CAD build for the part. Positions are in the model's coordinates, mm. A direction names the side the tool comes from. Round coordinates to 2 decimals unless told otherwise and drop trailing zeros. Loops run counter-clockwise (first coordinate to the right, second up) from the corner with the lowest first, then second, coordinate; pieces in that order, holes last. Notation, with made-up numbers: M -6,12 L 40,12 A24 ccw 40,46 Z; hole C 70.25,54.25 d1. An arc over 180 degrees is marked long. Use one line per item in the form item = value.
from build123d import *

# Parameters (mm, degrees)
SKETCH1_R           = 2
BOSS_EXTRUDE1_DEPTH = 2
CHAMFER1_SIZE       = 0.3
CUT_EXTRUDE1_DEPTH  = 1.5
CHAMFER2_SIZE       = 0.2
SKETCH3_R           = 1
BOSS_EXTRUDE2_DEPTH = 6
CHAMFER3_SIZE       = 0.2


with BuildPart() as part:
    # Sketch1 → Boss-Extrude1 (new body)
    with BuildSketch(Plane(origin=(0, 0, 0), x_dir=(1, 0, 0), z_dir=(0, 1, 0))):
        with Locations(Location((0, 0, 0), (0, 0, 270))):  # turned: the seam where the file's is
            Circle(SKETCH1_R)
    extrude(amount=BOSS_EXTRUDE1_DEPTH)

    # Chamfer1
    chamfer1_edges = [part.edges().sort_by_distance(p)[0] for p in [
        (0, 2, -2),
    ]]
    chamfer(chamfer1_edges, length=CHAMFER1_SIZE)

    # Sketch2 → Cut-Extrude1 (cut)
    with BuildSketch(Plane(origin=(0, 2, 0), x_dir=(1, 0, 0), z_dir=(0, 1, 0))):
        Polygon((1.154700538, 0), (0.577350269, 1), (-0.577350269, 1), (-1.154700538, 0), (-0.577350269, -1), (0.577350269, -1), align=None)
    extrude(amount=-CUT_EXTRUDE1_DEPTH, mode=Mode.SUBTRACT)

    # Chamfer2
    chamfer2_edges = [part.edges().sort_by_distance(p)[0] for p in [
        (0.866025404, 2, 0.5),
        (0.866025404, 2, -0.5),
        (0, 2, -1),
        (-0.866025404, 2, -0.5),
        (-0.866025404, 2, 0.5),
        (0, 2, 1),
    ]]
    chamfer(chamfer2_edges, length=CHAMFER2_SIZE)

    # Sketch3 → Boss-Extrude2 (add)
    with BuildSketch(Plane.XZ):
        with Locations(Location((0, 0, 0), (0, 0, 90))):  # turned: the seam where the file's is
            Circle(SKETCH3_R)
    extrude(amount=BOSS_EXTRUDE2_DEPTH)

    # Chamfer3
    chamfer3_edges = [part.edges().sort_by_distance(p)[0] for p in [
        (0, -6, -1),
    ]]
    chamfer(chamfer3_edges, length=CHAMFER3_SIZE)


solid = part.part
1. Tool access for faces 5 (the face through (0, -6, 0)), 6 (the face through (-0.86, 1.16, -0.51)), 7 (the face through (-1, 0, 1)): list every direction of +Z, -Z, +X, -X, +Y, -Y with a clear straight run to the whole face (end or side of a thin tool).
Completed:
face_5 = +Z, -Z, +X, -X, -Y
face_6 = +Y
face_7 = -Y
2. Cut at A-A on x = 0. Write the cut outline in (y, z).
Completed:
outline = M -6,-0.8 L -5.8,-1 L 0,-1 L 0,-2 L 1.7,-2 L 2,-1.7 L 2,-1.2 L 1.8,-1 L 0.5,-1 L 0.5,1 L 1.8,1 L 2,1.2 L 2,1.7 L 1.7,2 L 0,2 L 0,1 L -5.8,1 L -6,0.8 Z
3. Probe line 1 along Y through (x, z) = (-1.3, 0.3); line 2 along Z through (x, y) = (0.35, 1); line 3 along X through (y, z) = (1.25, 0.25). List the from-to ranges inside material, lowest first. Write a range as from..to.
Completed:
line_1 = 0..2
line_2 = -1.97..-1, 1..1.97
line_3 = -1.98..-1.01, 1.01..1.98
4. Drop flat-ended pins along their axis: P1, Ø2, axis at x = 0.5, y = -2, coming from the +Z side; P2, Ø0.6, axis at x = -0.5, z = 0, coming from the +Y side; P3, Ø1.5, axis at y = -1.5, z = -0.5, coming from the -X side. Give the stop position or say it passes through.
Completed:
P1 = 1
P2 = 0.5
P3 = -1
5. Pull direction Z, two halves, no side cores. Call faces 1 (the face through (0.86, 1.16, 0.51)), 2 (the face through (0.87, 1.16, -0.49)), 3 (the face through (1, -3, 0)), 4 (the face through (1, 2, 1)): +Z half, -Z half, draft (parallel to the pull), parting line (faces both ways), or undercut.
Completed:
face_1 = undercut
face_2 = undercut
face_3 = parting line
face_4 = draft
6. Cut at B-B on y = -0.25. Write the cut outline in (x, z).
Completed:
outline = C 0,0 d2
